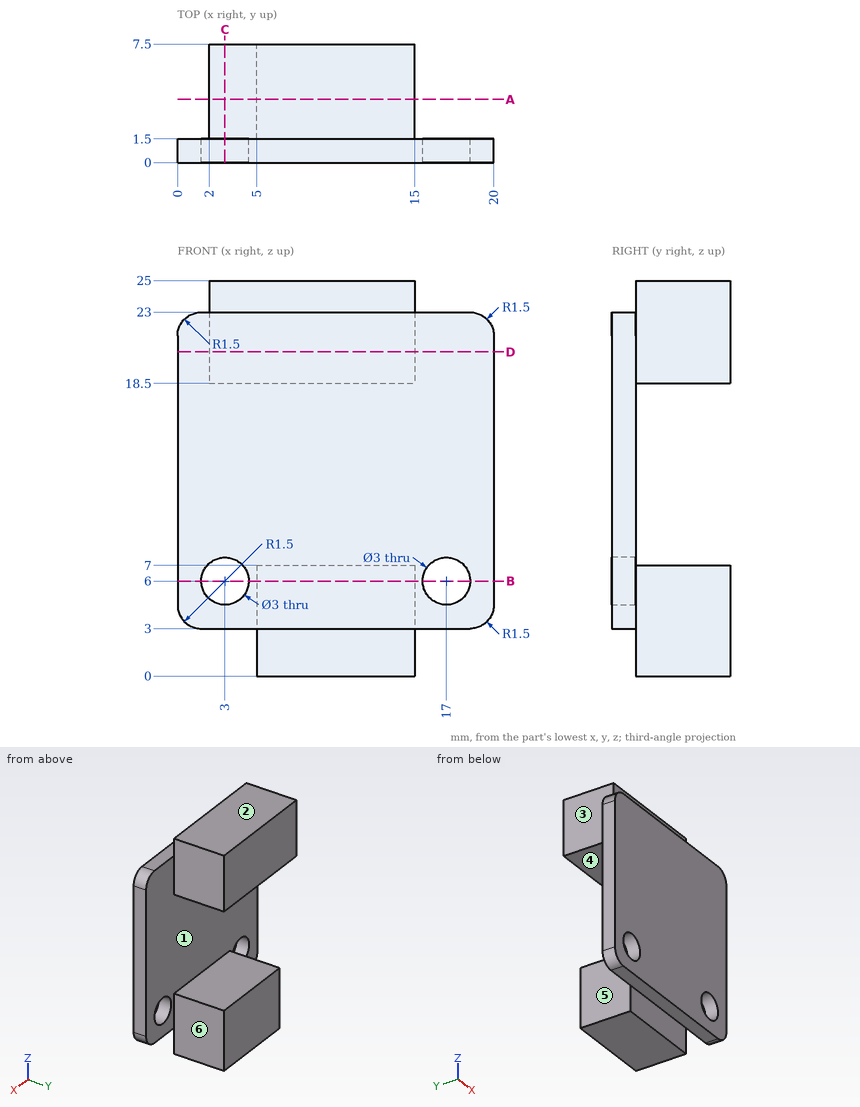
The figure shows three views and two pictorial views of one solid part (mm, origin at its lowest corner). Answer the questions. A direction names the side the tool comes from. Coordinates: 2 decimals unless noted, no trailing zeros. Write each loop counter-clockwise with the first axis right and the second up, starting at its lowest first coordinate (ties: lowest second). Pieces come first, ordered by that corner, then holes. Notation, with made-up numbers: (56, 85) -> (110, 85) arc R17 cw to (110, 95) -> close; hole circle Ø10 at (-28.5, 45). An arc over 180 degrees is marked (long way). Return JSON: item names as keys, results as strings.
(1) For a pull along Z with two mould halves and no side action, classify the marked faces 1, 2 and 3 as pulls with the +Z half, pulls with the -Z half, needs draft (parallel to the pull), parting line crosses it, or undercut.
Answers below:
{"face 1": "undercut", "face 2": "pulls with the +Z half", "face 3": "needs draft"}
(2) The part is cut by section D-D on z = 20.5. Give the vertices of the cut face in (x, y).
Answers below:
{"outline": "(0, 0) -> (20, 0) -> (20, 1.5) -> (15, 1.5) -> (15, 7.5) -> (2, 7.5) -> (2, 1.5) -> (0, 1.5) -> close"}
(3) The part is cut by section B-B on z = 6. Give the vertices of the cut face in (x, y), then the cut area to 3 significant figures.
Answers below:
{"outline": "(0, 0) -> (1.5, 0) -> (1.5, 1.5) -> (0, 1.5) -> close; (4.5, 0) -> (15.5, 0) -> (15.5, 1.5) -> (15, 1.5) -> (15, 7.5) -> (5, 7.5) -> (5, 1.5) -> (4.5, 1.5) -> close; (18.5, 0) -> (20, 0) -> (20, 1.5) -> (18.5, 1.5) -> close", "area": "81.0 mm^2"}
(4) The part is cut by section C-C on x = 3. Give the vertices of the cut face in (y, z).
Answers below:
{"outline": "(0, 3) -> (1.5, 3) -> (1.5, 4.5) -> (0, 4.5) -> close; (0, 7.5) -> (1.5, 7.5) -> (1.5, 18.5) -> (7.5, 18.5) -> (7.5, 25) -> (1.5, 25) -> (1.5, 23) -> (0, 23) -> close"}
(5) Each of these flat-tipped pins is pushed along its axis until it touches: P1, Ø0.8, axis at x = 13.5, y = 1, coming from the +Z side; P2, Ø1.5, axis at x = 8.5, z = 1.5, coming from the -Y side; P3, Ø1.8, axis at x = 3, z = 6, coming from the +Y side; P4, Ø1.8, axis at y = 4.5, z = 2.5, coming from the +X side. Where does it stop, or does it pass through?
Answers below:
{"P1": "z = 23", "P2": "y = 1.5", "P3": "through", "P4": "x = 15"}
(6) Consider line 1 along X through (y, z) = (0.9, 6); line 2 along Z through (x, y) = (5.5, 6.5); line 3 along Y through (x, z) = (7.25, 9.5). Determine where each line is inside the solid, lowest interval first. Write a range as from..to.
Answers below:
{"line 1": "0..1.5, 4.5..15.5, 18.5..20", "line 2": "0..7, 18.5..25", "line 3": "0..1.5"}
(7) Which of the six approach directions +Z, -Z, +X, -X, +Y, -Y give full straight-line access (tool end or side, diameter ignored) to the marked faces 4, 5 and 6?
Answers below:
{"face 4": "+X, -X, +Y", "face 5": "-Z, -X, +Y", "face 6": "+Z, -Z, +X, +Y"}
(8) The part is cut by section A-A on y = 4. Give the vertices of the cut face in (x, z), then the cut area to 4 significant figures.
Answers below:
{"outline": "(2, 18.5) -> (15, 18.5) -> (15, 25) -> (2, 25) -> close; (5, 0) -> (15, 0) -> (15, 7) -> (5, 7) -> close", "area": "154.5 mm^2"}
